from build123d import *

# Parameters (mm, degrees)
ESQUISSE1_W                = 130
ESQUISSE1_H                = 32
ESQUISSE1_R                = 1.5
BOSS_EXTRU_1_DEPTH         = 13
D_GAGEMENT_M31_D           = 3.4
D_GAGEMENT_M31_DEPTH       = 13
R_P_TITION_LIN_AIRE1_COUNT = 4
R_P_TITION_LIN_AIRE1_PITCH = 32.8


with BuildPart() as part:
    # Esquisse1 → Boss.-Extru.1 (new body)
    with BuildSketch(Plane.XY):
        with Locations((65, 16)):
            Rectangle(ESQUISSE1_W, ESQUISSE1_H)
        with Locations(Location((2.8, 26.3, 0), (0, 0, 180))):
            Circle(ESQUISSE1_R, mode=Mode.SUBTRACT)
        with Locations(Location((29, 26.3, 0), (0, 0, 180))):
            Circle(ESQUISSE1_R, mode=Mode.SUBTRACT)
        with Locations(Location((2.8, 5.7, 0), (0, 0, 180))):
            Circle(ESQUISSE1_R, mode=Mode.SUBTRACT)
        with Locations(Location((29, 5.7, 0), (0, 0, 180))):
            Circle(ESQUISSE1_R, mode=Mode.SUBTRACT)
    extrude(amount=BOSS_EXTRU_1_DEPTH)

    # Dégagement M31
    with Locations(Plane.XY.offset(13)):
        with Locations((2.8, 26.3), (29, 26.3), (2.8, 5.7), (29, 5.7)):
            d_gagement_m31 = Hole(D_GAGEMENT_M31_D / 2, depth=D_GAGEMENT_M31_DEPTH)

    # Répétition linéaire1: Dégagement M31 ×4
    with Locations(*[(i * R_P_TITION_LIN_AIRE1_PITCH, 0, 0) for i in range(1, R_P_TITION_LIN_AIRE1_COUNT)]):
        add(d_gagement_m31, mode=Mode.SUBTRACT)


solid = part.part
Verification items for the finished model (mm, model axes). Round coordinates to 2 decimals unless told otherwise and drop trailing zeros. Write each loop counter-clockwise with the first axis right and the second up, starting at its lowest first coordinate (ties: lowest second). Pieces come first, ordered by that corner, then holes.
(1) Section check A-A (x = 2.8). Enter the section's corners in (y, z).
Returned:
outline: (0, 0) - (4, 0) - (4, 13) - (0, 13) - close; (7.4, 0) - (24.6, 0) - (24.6, 13) - (7.4, 13) - close; (28, 0) - (32, 0) - (32, 13) - (28, 13) - close
(2) Section check B-B (z = 6). Give the number of separate pieces and of enclosed holes in the cut face, plus the area to 3 significant figures.
Returned:
separate pieces: 1
enclosed holes: 16
area: 4,010 mm2
(3) Mould release check, pull along X, two halves, no side actions. Record for faces 1 (the cylindrical face through (125.78, 26.81, 6.41)), 2 (the flat face through (130, 16, 6)), 3 (the flat face through (64, 16, 0)): pulls with the +X half, pulls with the -X half, needs draft (parallel to the pull), parting line crosses it, or undercut.
Returned:
face 1: undercut
face 2: pulls with the +X half
face 3: needs draft
(4) Material ranges on line 1 (Y direction, x = 29, z = 7.25); line 2 (Y direction, x = 28.5, z = 6.75), recorded low to high.
Returned:
line 1: y = 0 to 4, 7.4 to 24.6, 28 to 32
line 2: y = 0 to 4.08, 7.32 to 24.68, 27.92 to 32
(5) Depth check by flat-ended pin: pin 1 Ø2.5 at (x, y) = (29, 5.7) entering from -Z. Enter the tip coordinate at first touch or a pass-through.
Returned:
pin 1: passes through
